Read the model definition and answer for the solid it produces. Units are mm, in the model's axes. Coordinates: 2 decimals unless noted, no trailing zeros. Order: outer loops, then holes, each group sorted by start corner. A loop starts at its lowest first (then second) coordinate and runs counter-clockwise, first axis right, second up. Notation, with made-up numbers: (2.5, -9) -> (49.5, -9) arc R12 ccw to (49.5, -2) -> close; hole circle Ø9 at (-11, 60.5). An arc over 180 degrees is marked (long way). Return JSON: item names as keys, results as strings. Group by question number.
Autodesk Inventor part; units mm, degrees
ref_plane "YZ Plane" through (0, 0, 0) normal (1, 0, 0) x (0, 1, 0)
ref_plane "XZ Plane" through (0, 0, 0) normal (0, 1, 0) x (-1, 0, 0)
ref_plane "XY Plane" through (0, 0, 0) normal (0, 0, 1) x (1, 0, 0)
sketch "Sketch1" plane through (0, 0, 0) normal (0, 0, 1) x (1, 0, 0)
  line L0 (-40, 0) -> (-40, -29)
  line L1 (-39, -30) -> (39, -30)
  line L2 (40, -29) -> (40, 0)
  line L3 (100, -60) -> (102, -60)
  line L4 (103, -61) -> (103, -69)
  line L5 (102, -70) -> (-102, -70)
  line L6 (-103, -69) -> (-103, -61)
  line L7 (-102, -60) -> (-100, -60)
  line L8 (-60, 0) -> (-60, 3)
  line L9 (-60, 3) -> (-70, 3)
  line L10 (-70, 3) -> (-70, 0)
  line L11 (-90, 0) -> (-70, 0)
  line L12 (-60, 0) -> (-40, 0)
  line L13 (70, 0) -> (70, 3)
  line L14 (70, 3) -> (60, 3)
  line L15 (60, 3) -> (60, 0)
  line L16 (40, 0) -> (60, 0)
  line L17 (70, 0) -> (90, 0)
  arc A0 (-103, -69) -> (-102, -70) centre (-102, -69) ccw
  arc A1 (102, -70) -> (103, -69) centre (102, -69) ccw
  arc A2 (39, -30) -> (40, -29) centre (39, -29) ccw
  arc A3 (-40, -29) -> (-39, -30) centre (-39, -29) ccw
  line L18 (-90, -40) -> (-84, -40)
  line L19 (-84, -40) -> (-84, -50)
  line L20 (90, -40) -> (84, -40)
  line L21 (84, -40) -> (84, -50)
  line L22 (-43.5, -10) -> (-46.5, -10)
  line L23 (-46.5, -10) -> (-46.5, -20)
  line L24 (-46.5, -20) -> (-43.5, -20)
  line L25 (-43.5, -20) -> (-43.5, -10)
  line L26 (43.5, -10) -> (46.5, -10)
  line L27 (46.5, -10) -> (46.5, -20)
  line L28 (46.5, -20) -> (43.5, -20)
  line L29 (43.5, -20) -> (43.5, -10)
  line L30 (-46.5, -50) -> (-43.5, -50)
  line L31 (-43.5, -50) -> (-43.5, -60)
  line L32 (-43.5, -60) -> (-46.5, -60)
  line L33 (-46.5, -60) -> (-46.5, -50)
  line L34 (43.5, -50) -> (46.5, -50)
  line L35 (46.5, -50) -> (46.5, -60)
  line L36 (46.5, -60) -> (43.5, -60)
  line L37 (43.5, -60) -> (43.5, -50)
  line L38 (-5, -53) -> (5, -53)
  line L39 (5, -53) -> (5, -56)
  line L40 (5, -56) -> (-5, -56)
  line L41 (-5, -56) -> (-5, -53)
  line L42 (-100, -60) -> (-100, -20)
  line L43 (-100, -20) -> (-92, -20)
  line L44 (-90, -40) -> (-90, -50)
  line L45 (90, -40) -> (90, -50)
  line L46 (90, -50) -> (84, -50)
  line L47 (100, -60) -> (100, -20)
  line L48 (100, -20) -> (92, -20)
  line L49 (90, -18) -> (90, 0)
  line L50 (-90, 0) -> (-90, -18)
  arc A4 (-92, -20) -> (-90, -18) centre (-92, -18) ccw
  arc A5 (90, -18) -> (92, -20) centre (92, -18) ccw
  line L51 (-90, -50) -> (-84, -50)
  arc A6 (-102, -60) -> (-103, -61) centre (-102, -61) ccw
  arc A7 (103, -61) -> (102, -60) centre (102, -61) ccw
  point P0 (0, 0)
  point P1 (-40, -30)
  point P2 (40, -30)
  point P3 (103, -60)
  point P4 (103, -70)
  point P5 (-103, -70)
  point P6 (-103, -60)
  point P7 (-90, -20)
  point P8 (90, -20)
  dimension "d0" = 80
  dimension "d1" = 30
  dimension "d2" = 50
  dimension "d5" = 10
  dimension "d7" = 10
  dimension "d10" = 50
  dimension "d13" = 3
  dimension "d14" = 3
  dimension "d15" = 3
  dimension "d16" = 10
  dimension "d18" = 10
  dimension "d20" = 3
  dimension "d21" = 40
  dimension "d22" = 206
  dimension "d23" = 30
  dimension "d24" = 40
  dimension "d27" = 1
  dimension "d28" = 10
  dimension "d29" = 6
  dimension "d31" = 40
  dimension "d32" = 10
  dimension "d33" = 6
  dimension "d35" = 40
  dimension "d39" = 10
  dimension "d40" = 3
  dimension "d41" = 10
  dimension "d42" = 3
  dimension "d44" = 10
  dimension "d45" = 10
  dimension "d50" = 3
  dimension "d51" = 10
  dimension "d52" = 10
  dimension "d54" = 3
  dimension "d55" = 10
  dimension "d56" = 10
  dimension "d60" = 10
  dimension "d61" = 3
  dimension "d62" = 17
  dimension "d66" = 40
  dimension "d67" = 40
  dimension "d71" = 3.5
  dimension "d72" = 3.5
  dimension "d73" = 3.5
  dimension "d74" = 3.5
  dimension "d77" = 20
  dimension "d78" = 20
  dimension "d79" = 10
  dimension "d80" = 10
  dimension "d81" = 2
  dimension "d82" = 10
  dimension "d84" = 50
  dimension "d85" = 20
  dimension "d86" = 20
  dimension "d87" = 60
  dimension "d88" = 5
  dimension "d91" = 1
extrude "Extrusion7" add sketch "Sketch1" along normal blind 3
properties part number "OpenROV 2_3 Dev Bulkhead"
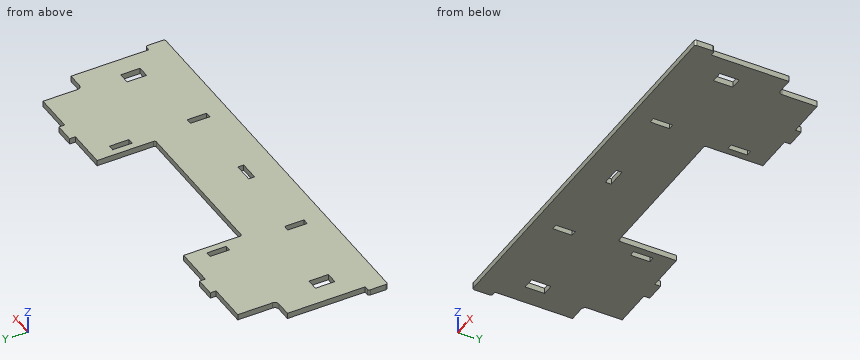
1. Find section D-D on z = 1.05. Give the number of separate pieces and of enclosed holes in the cut face, and give its area (3 significant figures).
2. Find section C-C on y = -42.5. Determine the outline of the cut face in (x, z).
3. Straight lines are drawn through the part: L1, parallel to X at y = -40.5, z = 0.3; L2, parallel to X at y = -15.5, z = 2.4; L3, parallel to Y at x = 1.5, z = 0.6. For each, find the intervals that lie inside material, in ascending order.
4. Find section A-A on x = 3. Determine the outline of the cut face in (y, z), and give its area (3 significant figures).
5. Given pin 1 (0.9 mm diameter, centred on y = -9, z = 2, fed in from -X); pin 2 (0.9 mm diameter, centred on y = -45, z = 1, fed in from -X); pin 3 (0.9 mm diameter, centred on x = -96, z = 2, fed in from +Y), each flat-ended and moving along its own axis, determine where each tip first touches the part or whether it passes through.
6. Find section B-B on y = -7.5. Determine the outline of the cut face in (x, z), and give its area (3 significant figures).
Result:
{
 "1": {"separate pieces": "1", "enclosed holes": "7", "area": "11,100 mm^2"},
 "2": {"outline": "(-100, 0) -> (-90, 0) -> (-90, 3) -> (-100, 3) -> close; (-84, 0) -> (84, 0) -> (84, 3) -> (-84, 3) -> close; (90, 0) -> (100, 0) -> (100, 3) -> (90, 3) -> close"},
 "3": {"L1": "-100 to -90, -84 to 84, 90 to 100", "L2": "-90 to -46.5, -43.5 to -40, 40 to 43.5, 46.5 to 90", "L3": "-70 to -56, -53 to -30"},
 "4": {"outline": "(-70, 0) -> (-56, 0) -> (-56, 3) -> (-70, 3) -> close; (-53, 0) -> (-30, 0) -> (-30, 3) -> (-53, 3) -> close", "area": "111 mm^2"},
 "5": {"pin 1": "x = -90", "pin 2": "x = -100", "pin 3": "y = -20"},
 "6": {"outline": "(-90, 0) -> (-40, 0) -> (-40, 3) -> (-90, 3) -> close; (40, 0) -> (90, 0) -> (90, 3) -> (40, 3) -> close", "area": "300 mm^2"}
}
